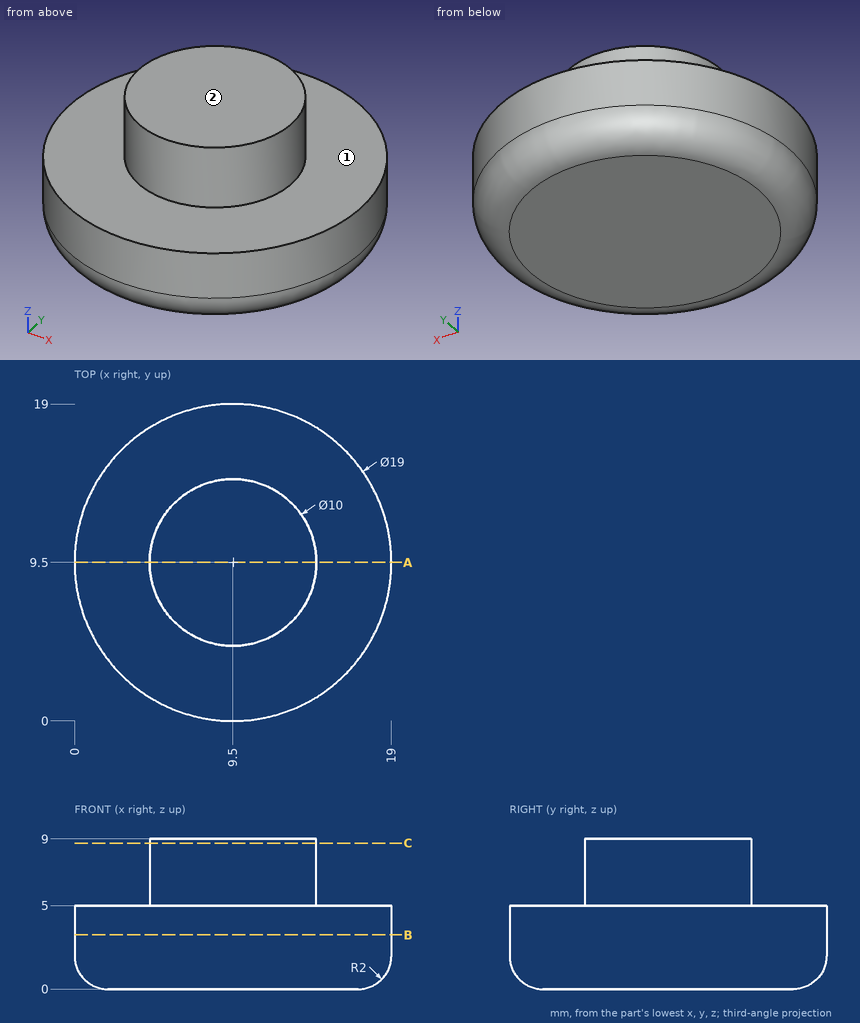
Geometry check sheet. Reference: drawing and pictorial views, mm from the part's lowest x, y, z. A direction names the side the tool comes from. Round coordinates to 2 decimals unless told otherwise and drop trailing zeros. Loops run counter-clockwise (first coordinate to the right, second up) from the corner with the lowest first, then second, coordinate; pieces in that order, holes last. Notation, with made-up numbers: (12.25, 63) - (59.25, 63) arc R11 cw to (59.25, 73) - close; hole circle Ø10 at (-0.5, 65). An arc over 180 degrees is marked (long way). Answer as CSV lines item,"result".
(1) Cross-section at A-A, the plane y = 9.5. Enter the section's corners in (x, z).
Output values:
outline,"(0, 2) arc R2 ccw to (2, 0) - (17, 0) arc R2 ccw to (19, 2) - (19, 5) - (14.5, 5) - (14.5, 9) - (4.5, 9) - (4.5, 5) - (0, 5) - close"
(2) Material ranges on line 1 along Y through (x, z) = (9.75, 3.5); line 2 along Z through (x, y) = (3.5, 6.75); line 3 along Y through (x, z) = (8.75, 8.25), recorded low to high.
Output values:
line 1,"y = 0 to 19"
line 2,"z = 0 to 5"
line 3,"y = 4.56 to 14.44"
(3) Depth check by flat-ended pin: pin 1 Ø5 at (x, z) = (14, 6) entering from -Y; pin 2 Ø4 at (y, z) = (14, 5.5) entering from +X; pin 3 Ø4 at (y, z) = (12.5, 4.5) entering from -X. Enter the tip coordinate at first touch or a pass-through.
Output values:
pin 1,"stops at y = 0.26"
pin 2,"stops at x = 18.65"
pin 3,"stops at x = 0.05"
(4) Set-up check for the marked faces 1 and 2: record each of +Z, -Z, +X, -X, +Y, -Y from which the full face is reachable in a straight line by a thin tool's end or side.
Output values:
face 1,"+Z"
face 2,"+Z, +X, -X, +Y, -Y"
(5) Cross-section at C-C, the plane z = 8.75. Enter the section's corners in (x, y), and give its area (3 significant figures).
Output values:
outline,"circle Ø10 at (9.5, 9.5)"
area,"78.5 mm²"
(6) Cross-section at B-B, the plane z = 3.25. Enter the section's corners in (x, y).
Output values:
outline,"circle Ø19 at (9.5, 9.5)"
